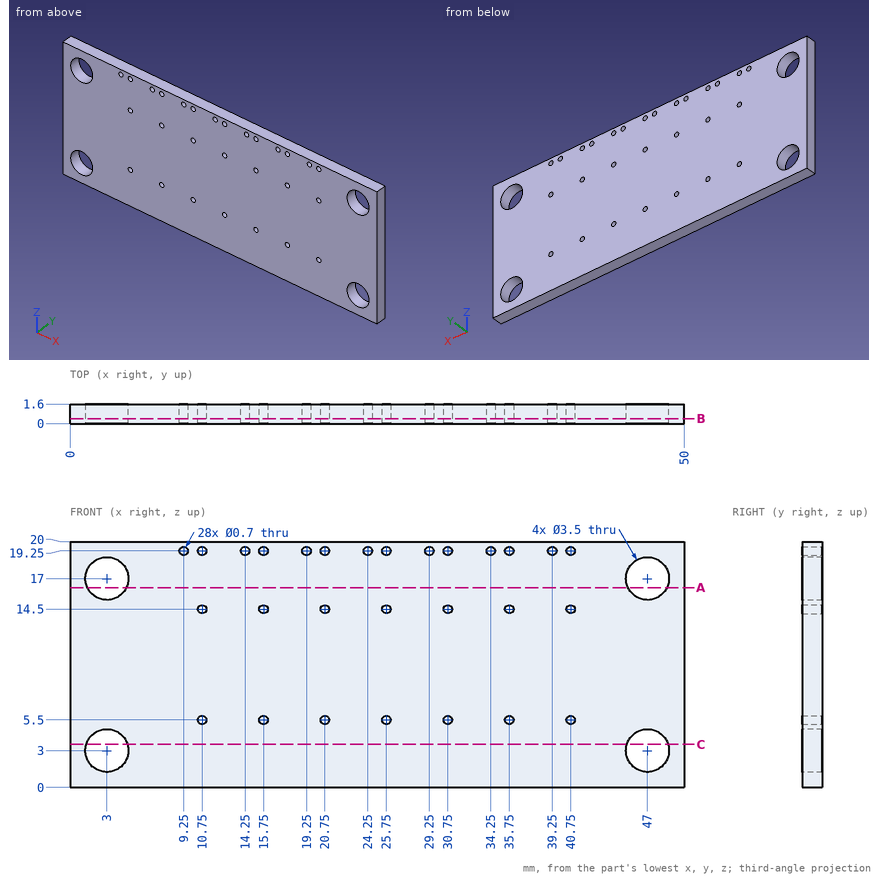
Answer from the drawing. Dimensions are ordinates in mm from the lowest x, y and z of the part. Coordinates: 2 decimals unless noted, no trailing zeros. Loops run counter-clockwise (first coordinate to the right, second up) from the corner with the lowest first, then second, coordinate; pieces in that order, holes last. Notation, with made-up numbers: (21, 70) -> (74, 70) arc R12 cw to (74, 82) -> close; hole circle Ø4 at (4, 42). An arc over 180 degrees is marked (long way). Return JSON: item names as keys, results as strings.
Item 1: Find section A-A (z = 16.25). Determine the outline of the cut face in (x, y).
Answers:
{"outline": "(0, 0) -> (1.42, 0) -> (1.42, 1.6) -> (0, 1.6) -> close; (4.58, 0) -> (45.42, 0) -> (45.42, 1.6) -> (4.58, 1.6) -> close; (48.58, 0) -> (50, 0) -> (50, 1.6) -> (48.58, 1.6) -> close"}
Item 2: Flat-ended cylindrical pins translate along their axes: P1, Ø5.5, axis at x = 3, z = 17, coming from the -Y side; P2, Ø3, axis at x = 3, z = 3, coming from the -Y side. Find the tip coordinate at first contact, or state that the pin passes through.
Answers:
{"P1": "stops at y = 0", "P2": "passes through"}
Item 3: Find section C-C (z = 3.5). Determine the outline of the cut face in (x, y).
Answers:
{"outline": "(0, 0) -> (1.32, 0) -> (1.32, 1.6) -> (0, 1.6) -> close; (4.68, 0) -> (45.32, 0) -> (45.32, 1.6) -> (4.68, 1.6) -> close; (48.68, 0) -> (50, 0) -> (50, 1.6) -> (48.68, 1.6) -> close"}
Item 4: Find the intervals of material crossed by probe 1 along X at (y, z) = (0.55, 3); probe 2 along Z at (x, y) = (35.75, 0.9); probe 3 along Z at (x, y) = (47, 0.7), in increasing order.
Answers:
{"probe 1": "x = 0 to 1.25, 4.75 to 45.25, 48.75 to 50", "probe 2": "z = 0 to 5.15, 5.85 to 14.15, 14.85 to 18.9, 19.6 to 20", "probe 3": "z = 0 to 1.25, 4.75 to 15.25, 18.75 to 20"}
Item 5: Find section B-B (y = 0.4). Count the separate pieces of the cut face and the enclosed holes in it, plus the area to 3 significant figures.
Answers:
{"separate pieces": "1", "enclosed holes": "32", "area": "951 mm2"}
